from build123d import *

# Parameters (mm, degrees)
SKETCH1_R           = 24.375
BOSS_EXTRUDE1_DEPTH = 54.25
CHAMFER1_SIZE       = 9.25
CHAMFER1_SIZE2      = 3.125
CHAMFER2_SIZE       = 8
CUT_EXTRUDE1_DEPTH  = 10
SKETCH3_R           = 7
BOSS_EXTRUDE2_DEPTH = 5
SKETCH4_R           = 3
BOSS_EXTRUDE3_DEPTH = 18


with BuildPart() as part:
    # Sketch1 → Boss-Extrude1 (new body)
    with BuildSketch(Plane(origin=(0, 0, 0), x_dir=(1, 0, 0), z_dir=(0, 1, 0))):
        with Locations(Location((0, 0, 0), (0, 0, 270))):
            Circle(SKETCH1_R)
    extrude(amount=BOSS_EXTRUDE1_DEPTH)

    # Chamfer1
    chamfer1_edges = [part.edges().sort_by_distance(p)[0] for p in [
        (0, 54.25, -24.375),
    ]]
    chamfer1_side = [part.faces().sort_by_distance(p)[0] for p in [
        (0, 27.125, -24.375),
    ]]
    chamfer(chamfer1_edges, length=CHAMFER1_SIZE, length2=CHAMFER1_SIZE2, reference=chamfer1_side[0])

    # Chamfer2
    chamfer2_edges = [part.edges().sort_by_distance(p)[0] for p in [
        (0, 0, -24.375),
    ]]
    chamfer(chamfer2_edges, length=CHAMFER2_SIZE)

    # Sketch2 → Cut-Extrude1 (cut)
    with BuildSketch(Plane.XZ):
        with BuildLine():
            Line((-3.752441842, -18.058791036), (-3.127941128, -14.70103845))
            ThreePointArc((-3.127941128, -14.70103845), (-3.399785699, -13.030905705), (-4.673081087, -11.916472345))
            ThreePointArc((-4.673081087, -11.916472345), (-7.523651229, -10.355417528), (-9.889177203, -8.126756686))
            ThreePointArc((-9.889177203, -8.126756686), (-11.342536225, -7.260159658), (-13.014931448, -7.517719508))
            Line((-13.014931448, -7.517719508), (-16.015362591, -9.149257594))
            ThreePointArc((-16.015362591, -9.149257594), (-17.266321132, -10.825132639), (-16.80622135, -12.865172499))
            ThreePointArc((-16.80622135, -12.865172499), (-12.440537552, -17.122930967), (-7.04209813, -19.959223267))
            ThreePointArc((-7.04209813, -19.959223267), (-4.959726276, -19.766397177), (-3.752441842, -18.058791036))
        make_face()
        with BuildLine():
            Line((-18.33449919, -2.011689062), (-14.94810538, -1.568021924))
            ThreePointArc((-14.94810538, -1.568021924), (-13.443719342, -0.793382972), (-12.777300147, 0.761971751))
            ThreePointArc((-12.777300147, 0.761971751), (-12.173523409, 3.955417528), (-10.784928719, 6.893860495))
            ThreePointArc((-10.784928719, 6.893860495), (-10.409858605, 8.543880272), (-11.171611124, 10.054832276))
            Line((-11.171611124, 10.054832276), (-13.650480266, 12.404238871))
            ThreePointArc((-13.650480266, 12.404238871), (-15.630899596, 13.076097273), (-17.428914147, 12.008109392))
            ThreePointArc((-17.428914147, 12.008109392), (-20.129212597, 6.540377643), (-21.158477347, 0.529694131))
            ThreePointArc((-21.158477347, 0.529694131), (-20.331600546, -1.391172651), (-18.33449919, -2.011689062))
        make_face()
        with BuildLine():
            Line((3.752441842, -18.058791036), (3.127941128, -14.70103845))
            ThreePointArc((3.127941128, -14.70103845), (3.399785699, -13.030905705), (4.673081087, -11.916472345))
            ThreePointArc((4.673081087, -11.916472345), (7.523651229, -10.355417528), (9.889177203, -8.126756686))
            ThreePointArc((9.889177203, -8.126756686), (11.342536225, -7.260159658), (13.014931448, -7.517719508))
            Line((13.014931448, -7.517719508), (16.015362591, -9.149257594))
            ThreePointArc((16.015362591, -9.149257594), (17.266321132, -10.825132639), (16.80622135, -12.865172499))
            ThreePointArc((16.80622135, -12.865172499), (12.440537552, -17.122930967), (7.04209813, -19.959223267))
            ThreePointArc((7.04209813, -19.959223267), (4.959726276, -19.766397177), (3.752441842, -18.058791036))
        make_face()
        with BuildLine():
            Line((-7.578901824, 16.815498821), (-6.110496064, 13.731947606))
            ThreePointArc((-6.110496064, 13.731947606), (-4.908889789, 12.540568062), (-3.223724689, 12.387396786))
            ThreePointArc((-3.223724689, 12.387396786), (0, 12.8), (3.223724689, 12.387396786))
            ThreePointArc((3.223724689, 12.387396786), (4.908889789, 12.540568062), (6.110496064, 13.731947606))
            Line((6.110496064, 13.731947606), (7.578901824, 16.815498821))
            ThreePointArc((7.578901824, 16.815498821), (7.605893907, 18.906605194), (6.034560021, 20.286592244))
            ThreePointArc((6.034560021, 20.286592244), (0, 21.16510665), (-6.034560021, 20.286592244))
            ThreePointArc((-6.034560021, 20.286592244), (-7.605893907, 18.906605194), (-7.578901824, 16.815498821))
        make_face()
        with BuildLine():
            Line((13.650480266, 12.404238871), (11.171611124, 10.054832276))
            ThreePointArc((11.171611124, 10.054832276), (10.409858605, 8.543880272), (10.784928719, 6.893860495))
            ThreePointArc((10.784928719, 6.893860495), (12.173523409, 3.955417528), (12.777300147, 0.761971751))
            ThreePointArc((12.777300147, 0.761971751), (13.443719342, -0.793382972), (14.94810538, -1.568021924))
            Line((14.94810538, -1.568021924), (18.33449919, -2.011689062))
            ThreePointArc((18.33449919, -2.011689062), (20.331600546, -1.391172651), (21.158477347, 0.529694131))
            ThreePointArc((21.158477347, 0.529694131), (20.129212597, 6.540377643), (17.428914147, 12.008109392))
            ThreePointArc((17.428914147, 12.008109392), (15.630899596, 13.076097273), (13.650480266, 12.404238871))
        make_face()
    extrude(amount=-CUT_EXTRUDE1_DEPTH, mode=Mode.SUBTRACT)

    # Sketch3 → Boss-Extrude2 (add)
    with BuildSketch(Plane(origin=(0, 0, 0), x_dir=(-1, 0, 0), z_dir=(0, -1, 0))):
        with Locations(Location((0, 0, 0), (0, 0, 270))):
            Circle(SKETCH3_R)
    extrude(amount=BOSS_EXTRUDE2_DEPTH)

    # Sketch4 → Boss-Extrude3 (add)
    with BuildSketch(Plane(origin=(0, 54.25, 0), x_dir=(1, 0, 0), z_dir=(0, 1, 0))):
        with Locations(Location((0, 0, 0), (0, 0, 270))):
            Circle(SKETCH4_R)
    extrude(amount=BOSS_EXTRUDE3_DEPTH)


solid = part.part
Design review of the part built by this model. Coordinates are the model's own, in mm. Round coordinates to 2 decimals unless told otherwise and drop trailing zeros. Write each loop counter-clockwise with the first axis right and the second up, starting at its lowest first coordinate (ties: lowest second). Pieces come first, ordered by that corner, then holes. Notation, with made-up numbers: (84, -28.5) - (133, -28.5) arc R30 cw to (133, 2.5) - close; hole circle Ø5 at (30.5, -1.5). An arc over 180 degrees is marked (long way). Use a Markdown table: item, result. Add a question column.
1. We need section B-B (y = 61.5). State the section outline as (x, z) points.
2. Wall thickness on probe 1 along X at (y, z) = (7, -0.5); probe 2 along Y at (x, z) = (12.5, -5); probe 3 along Y at (x, z) = (7, -12): over which ranges is each line inside the solid? List them lowest first.
3. Mouldability with a two-part tool opening along X and no side actions: class faces 1 (the face through (-6.855, 4.93, 15.295)), 2 (the face through (-13, 53.8, -17)) as +X half, -X half, draft (parallel to the pull), parting line (faces both ways), or undercut.
4. We need section A-A (x = 0). State the section outline as (y, z) points (3 decimals), then the cut area to 3 significant figures.
5. We need section C-C (y = 16). State the section outline as (x, z) points (3 decimals), then the cut area to 3 significant figures.
6. Clearance check with flat-ended pins moving along their axes: pin 1 (5 mm diameter, centred on x = 12.5, z = -3.5, fed in from -Y); pin 2 (6 mm diameter, centred on y = 16.5, z = -8.5, fed in from +X); pin 3 (10 mm diameter, centred on x = -16.5, y = 52, fed in from +Z). State where each tip first meets the part, or that it passes through.
Output:
| question | item | result |
|---|---|---|
| 1 | outline | circle Ø6 at (0, 0) |
| 2 | probe 1 | x = -23.37 to -20.96, -13.21 to 13.21, 20.96 to 23.37 |
| 2 | probe 2 | y = 0 to 54.25 |
| 2 | probe 3 | y = 10 to 54.25 |
| 3 | face 1 | undercut |
| 3 | face 2 | parting line |
| 4 | outline | (-5, -7) - (0, -7) - (0, -16.375) - (8, -24.375) - (45, -24.375) - (54.25, -21.25) - (54.25, -3) - (72.25, -3) - (72.25, 3) - (54.25, 3) - (54.25, 21.25) - (45, 24.375) - (8, 24.375) - (4.79, 21.165) - (10, 21.165) - (10, 12.8) - (0, 12.8) - (0, 7) - (-5, 7) - close |
| 4 | area | 2,660 mm2 |
| 5 | outline | circle Ø48.75 at (0, 0) |
| 5 | area | 1,870 mm2 |
| 6 | pin 1 | stops at y = 0 |
| 6 | pin 2 | stops at x = 23.75 |
| 6 | pin 3 | stops at z = 19.35 |
